Read the model definition and answer for the solid it produces. Units are mm, in the model's axes. A direction names the side the tool comes from. Give positions to 0.01 mm unless a question says otherwise; leave off trailing zeros. Order: outer loops, then holes, each group sorted by start corner. A loop starts at its lowest first (then second) coordinate and runs counter-clockwise, first axis right, second up. Notation, with made-up numbers: (78, -19.75) - (89, -19.75) arc R22 ccw to (89, 8.25) - close; hole circle Ø10 at (37.5, -33). An arc over 180 degrees is marked (long way). Write item = value, one per line.
```python
from build123d import *

# Parameters (mm, degrees)
SKETCH1_R           = 1.5
BOSS_EXTRUDE1_DEPTH = 3
SKETCH2_W           = 26.5
SKETCH2_H           = 13.12704922
BOSS_EXTRUDE2_DEPTH = 3
SKETCH3_R           = 1.5
CUT_EXTRUDE1_DEPTH  = 10
SKETCH4_R           = 1.5
CUT_EXTRUDE2_DEPTH  = 10
BOSS_EXTRUDE4_START = -4
SKETCH6_R           = 1.5
SKETCH6_W           = 26.5
SKETCH6_H           = 25.74798773
BOSS_EXTRUDE4_DEPTH = 4
SKETCH9_R           = 1.5
CUT_EXTRUDE3_DEPTH  = 6
CUT_EXTRUDE4_DEPTH  = 14
SKETCH11_R          = 1.5
CUT_EXTRUDE5_DEPTH  = 14
SKETCH12_W          = 9.439157555
SKETCH12_H          = 13.291874924
CUT_EXTRUDE6_DEPTH  = 10
BOSS_EXTRUDE5_START = -6
SKETCH14_R          = 1.5
SKETCH14_R_2        = 1.624180029
SKETCH14_W          = 10
SKETCH14_H          = 12.873993865
SKETCH14_R_3        = 1.585240738
BOSS_EXTRUDE5_DEPTH = 6
SKETCH15_W          = 23.25
SKETCH15_H          = 10.234024539
CUT_EXTRUDE7_DEPTH  = 3
FILLET2_R           = 10
FILLET4_R           = 10
SKETCH16_W          = 26.5
SKETCH16_H          = 25.74798773
SKETCH16_H_2        = 10.370938511
SKETCH16_W_2        = 9.439157555
SKETCH16_H_3        = 13.291874924
BOSS_EXTRUDE6_DEPTH = 4
FILLET5_R           = 10


with BuildPart() as part:
    # Sketch1 → Boss-Extrude1 (new body)
    with BuildSketch(Plane(origin=(0, 0, 0), x_dir=(1, 0, 0), z_dir=(0, 1, 0))):
        Polygon((-5, -5), (41.5, -5), (41.5, 64.6), (31.5, 64.6), (-5, 56.73), align=None)
        Polygon((31.5, 54.48), (31.5, 5.234024539), (5, 5.234024539), (5, 56.73), align=None, mode=Mode.SUBTRACT)
        with Locations(Location((0, 0, 0), (0, 0, 270))):
            Circle(SKETCH1_R, mode=Mode.SUBTRACT)
        with Locations(Location((0, 51.73, 0), (0, 0, 270))):
            Circle(SKETCH1_R, mode=Mode.SUBTRACT)
        with Locations(Location((36.5, 59.6, 0), (0, 0, 270))):
            Circle(SKETCH1_R, mode=Mode.SUBTRACT)
        with Locations(Location((36.5, 11.18, 0), (0, 0, 270))):
            Circle(SKETCH1_R, mode=Mode.SUBTRACT)
        with Locations(Location((36.5, 49.6, 0), (0, 0, 270))):
            Circle(SKETCH1_R, mode=Mode.SUBTRACT)
    extrude(amount=BOSS_EXTRUDE1_DEPTH)

    # Sketch2 → Boss-Extrude2 (add)
    with BuildSketch(Plane(origin=(0, 3, 0), x_dir=(1, 0, 0), z_dir=(0, 1, 0))):
        with Locations((18.25, 37.545536879)):
            Rectangle(SKETCH2_W, SKETCH2_H)
        Polygon((5, 56.73), (5, 49.867078553), (31.5, 54.48), align=None)
    extrude(amount=-BOSS_EXTRUDE2_DEPTH)

    # Sketch3 → Cut-Extrude1 (cut)
    with BuildSketch(Plane(origin=(0, 3, 0), x_dir=(1, 0, 0), z_dir=(0, 1, 0))):
        with Locations(Location((10, 0, 0), (0, 0, 270))):
            Circle(SKETCH3_R)
    extrude(amount=-CUT_EXTRUDE1_DEPTH, mode=Mode.SUBTRACT)

    # Sketch4 → Cut-Extrude2 (cut)
    with BuildSketch(Plane(origin=(0, 3, 0), x_dir=(1, 0, 0), z_dir=(0, 1, 0))):
        with Locations(Location((0, 8, 0), (0, 0, 270))):
            Circle(SKETCH4_R)
    extrude(amount=-CUT_EXTRUDE2_DEPTH, mode=Mode.SUBTRACT)

    # Sketch6 → Boss-Extrude4 (add)
    # profile 1 of 3: a face of its own
    with BuildSketch(Plane(origin=(0, 3, 0), x_dir=(1, 0, 0), z_dir=(0, 1, 0)).offset(BOSS_EXTRUDE4_START)):
        Polygon((238, 64.6), (41.5, 64.6), (41.5, 29.8), (121.5, 49.6), (201.5, 29.8), (201.5, 56.73), align=None)
    # profile 2 of 3: a face of its own
    with BuildSketch(Plane(origin=(0, 3, 0), x_dir=(1, 0, 0), z_dir=(0, 1, 0)).offset(BOSS_EXTRUDE4_START)):
        Polygon((31.5, 64.6), (-5, 56.73), (-5, -5), (41.5, -5), (41.5, 29.8), (41.5, 64.6), align=None)
        with Locations(Location((0, 0, 0), (0, 0, 270))):
            Circle(SKETCH6_R, mode=Mode.SUBTRACT)
        with Locations(Location((10, 0, 0), (0, 0, 270))):
            Circle(SKETCH6_R, mode=Mode.SUBTRACT)
        with Locations(Location((0, 8, 0), (0, 0, 270))):
            Circle(SKETCH6_R, mode=Mode.SUBTRACT)
        with Locations(Location((36.5, 11.18, 0), (0, 0, 270))):
            Circle(SKETCH6_R, mode=Mode.SUBTRACT)
        with Locations((18.25, 18.108018404)):
            Rectangle(SKETCH6_W, SKETCH6_H, mode=Mode.SUBTRACT)
        Polygon((31.5, 44.109061489), (5, 44.109061489), (5, 49.867078553), (31.5, 54.48), align=None, mode=Mode.SUBTRACT)
        with Locations(Location((0, 51.73, 0), (0, 0, 270))):
            Circle(SKETCH6_R, mode=Mode.SUBTRACT)
        with Locations(Location((36.5, 49.6, 0), (0, 0, 270))):
            Circle(SKETCH6_R, mode=Mode.SUBTRACT)
        with Locations(Location((36.5, 59.6, 0), (0, 0, 270))):
            Circle(SKETCH6_R, mode=Mode.SUBTRACT)
    # profile 3 of 3: a face of its own
    with BuildSketch(Plane(origin=(0, 3, 0), x_dir=(1, 0, 0), z_dir=(0, 1, 0)).offset(BOSS_EXTRUDE4_START)):
        Polygon((248, 64.6), (238, 64.6), (201.5, 56.73), (201.5, -5), (248, -5), align=None)
        with Locations(Location((206.5, 8, 0), (0, 0, 270))):
            Circle(SKETCH6_R, mode=Mode.SUBTRACT)
        with Locations(Location((206.5, 0, 0), (0, 0, 270))):
            Circle(SKETCH6_R, mode=Mode.SUBTRACT)
        with Locations(Location((216.5, 0, 0), (0, 0, 270))):
            Circle(SKETCH6_R, mode=Mode.SUBTRACT)
        with Locations(Location((243, 11.18, 0), (0, 0, 270))):
            Circle(SKETCH6_R, mode=Mode.SUBTRACT)
        with Locations(Location((243, 49.6, 0), (0, 0, 270))):
            Circle(SKETCH6_R, mode=Mode.SUBTRACT)
        with Locations(Location((243, 59.6, 0), (0, 0, 270))):
            Circle(SKETCH6_R, mode=Mode.SUBTRACT)
        with Locations(Location((206.5, 51.73, 0), (0, 0, 270))):
            Circle(SKETCH6_R, mode=Mode.SUBTRACT)
        with Locations((224.75, 18.108018404)):
            Rectangle(SKETCH6_W, SKETCH6_H, mode=Mode.SUBTRACT)
        Polygon((238, 54.48), (238, 44.109061489), (211.5, 44.109061489), (211.5, 49.867078553), align=None, mode=Mode.SUBTRACT)
    extrude(amount=BOSS_EXTRUDE4_DEPTH)

    # Sketch9 → Cut-Extrude3 (cut)
    with BuildSketch(Plane(origin=(0, 3, 0), x_dir=(1, 0, 0), z_dir=(0, 1, 0))):
        with Locations(Location((61.5, 49.6, 0), (0, 0, 270))):
            Circle(SKETCH9_R)
        with Locations(Location((181.5, 49.6, 0), (0, 0, 270))):
            Circle(SKETCH9_R)
    extrude(amount=-CUT_EXTRUDE3_DEPTH, mode=Mode.SUBTRACT)

    # Sketch10 → Cut-Extrude4 (cut)
    with BuildSketch(Plane(origin=(0, 3, 0), x_dir=(1, 0, 0), z_dir=(0, 1, 0))):
        Polygon((79.758586054, 59.447076053), (79.758586054, 45.354236602), (102.023308671, 51.934500024), (102.023308671, 55.399132807), align=None)
        Polygon((140.976691329, 51.934500024), (140.976691329, 55.399132807), (163.241413946, 59.447076053), (163.241413946, 45.354236602), align=None)
    extrude(amount=-CUT_EXTRUDE4_DEPTH, mode=Mode.SUBTRACT)

    # Sketch11 → Cut-Extrude5 (cut)
    with BuildSketch(Plane(origin=(0, 3, 0), x_dir=(1, 0, 0), z_dir=(0, 1, 0))):
        with Locations(Location((71.5, 49.6, 0), (0, 0, 270))):
            Circle(SKETCH11_R)
        with Locations(Location((171.5, 49.6, 0), (0, 0, 270))):
            Circle(SKETCH11_R)
    extrude(amount=-CUT_EXTRUDE5_DEPTH, mode=Mode.SUBTRACT)

    # Sketch12 → Cut-Extrude6 (cut)
    with BuildSketch(Plane(origin=(0, 3, 0), x_dir=(1, 0, 0), z_dir=(0, 1, 0))):
        with Locations((193.819806215, 48.516488721)):
            Rectangle(SKETCH12_W, SKETCH12_H)
        with Locations((49.180193786, 48.516488721)):
            Rectangle(SKETCH12_W, SKETCH12_H)
    extrude(amount=-CUT_EXTRUDE6_DEPTH, mode=Mode.SUBTRACT)

    # Sketch14 → Boss-Extrude5 (add)
    # profile 1 of 6: a face of its own
    with BuildSketch(Plane(origin=(0, 3, 0), x_dir=(1, 0, 0), z_dir=(0, 1, 0)).offset(BOSS_EXTRUDE5_START)):
        Polygon((5, 18.108018404), (-5, 18.108018404), (-5, -5), (5, -5), (18.25, -5), (18.25, 5.234024539), (5, 5.234024539), align=None)
        with Locations(Location((0, 0, 0), (0, 0, 270))):
            Circle(SKETCH14_R, mode=Mode.SUBTRACT)
        with Locations(Location((10, 0, 0), (0, 0, 270))):
            Circle(SKETCH14_R, mode=Mode.SUBTRACT)
        with Locations(Location((0, 8, 0), (0, 0, 270))):
            Circle(SKETCH14_R_2, mode=Mode.SUBTRACT)
    # profile 2 of 6: a face of its own
    with BuildSketch(Plane(origin=(0, 3, 0), x_dir=(1, 0, 0), z_dir=(0, 1, 0)).offset(BOSS_EXTRUDE5_START)):
        Polygon((31.5, 5.234024539), (18.25, 5.234024539), (18.25, -5), (31.5, -5), (41.5, -5), (41.5, 5.234024539), align=None)
    # profile 3 of 6: a face of its own
    with BuildSketch(Plane(origin=(0, 3, 0), x_dir=(1, 0, 0), z_dir=(0, 1, 0)).offset(BOSS_EXTRUDE5_START)):
        with Locations((36.5, 11.671021472)):
            Rectangle(SKETCH14_W, SKETCH14_H)
        with Locations(Location((36.5, 11.18, 0), (0, 0, 270))):
            Circle(SKETCH14_R_3, mode=Mode.SUBTRACT)
    # profile 4 of 6: a face of its own
    with BuildSketch(Plane(origin=(0, 3, 0), x_dir=(1, 0, 0), z_dir=(0, 1, 0)).offset(BOSS_EXTRUDE5_START)):
        with Locations((243, 11.671021472)):
            Rectangle(SKETCH14_W, SKETCH14_H)
        with Locations(Location((243, 11.18, 0), (0, 0, 270))):
            Circle(SKETCH14_R, mode=Mode.SUBTRACT)
    # profile 5 of 6: a face of its own
    with BuildSketch(Plane(origin=(0, 3, 0), x_dir=(1, 0, 0), z_dir=(0, 1, 0)).offset(BOSS_EXTRUDE5_START)):
        Polygon((248, -5), (248, 5.234024539), (238, 5.234024539), (224.75, 5.234024539), (224.75, -5), (238, -5), align=None)
    # profile 6 of 6: a face of its own
    with BuildSketch(Plane(origin=(0, 3, 0), x_dir=(1, 0, 0), z_dir=(0, 1, 0)).offset(BOSS_EXTRUDE5_START)):
        Polygon((224.75, -5), (224.75, 5.234024539), (211.5, 5.234024539), (211.5, 18.108018404), (201.5, 18.108018404), (201.5, -5), (211.5, -5), align=None)
        with Locations(Location((206.5, 0, 0), (0, 0, 270))):
            Circle(SKETCH14_R, mode=Mode.SUBTRACT)
        with Locations(Location((216.5, 0, 0), (0, 0, 270))):
            Circle(SKETCH14_R, mode=Mode.SUBTRACT)
        with Locations(Location((206.5, 8, 0), (0, 0, 270))):
            Circle(SKETCH14_R, mode=Mode.SUBTRACT)
    extrude(amount=BOSS_EXTRUDE5_DEPTH)

    # Sketch15 → Cut-Extrude7 (cut)
    with BuildSketch(Plane(origin=(0, -3, 0), x_dir=(-1, 0, 0), z_dir=(0, -1, 0))):
        with Locations((-29.875, 0.117012269)):
            Rectangle(SKETCH15_W, SKETCH15_H)
        with Locations((-236.375, 0.117012269)):
            Rectangle(SKETCH15_W, SKETCH15_H)
    extrude(amount=-CUT_EXTRUDE7_DEPTH, mode=Mode.SUBTRACT)

    # Fillet2
    # the kernel refuses this fillet: 10 mm, written as the material it adds along each edge
    with BuildSketch(Plane(origin=(224.75, 0, 5), x_dir=(1, 0, 0), z_dir=(0, 0, -1)), Plane(origin=(18.25, 0, 5), x_dir=(1, 0, 0), z_dir=(0, 0, -1))) as fillet2_piece_1:
        with BuildLine():
            CenterArc((7.141428429, 10), FILLET2_R, 224.427004001, 45.572995999)
            Line((0, 3), (0, 0))
            Line((0, 0), (7.141428429, 0))
        make_face()
    extrude(amount=10.234024539)
    with BuildSketch(Plane(origin=(238, 0, -5.234024539), x_dir=(0, -1, 0), z_dir=(1, 0, 0)), Plane(origin=(31.5, 0, -5.234024539), x_dir=(0, -1, 0), z_dir=(1, 0, 0))) as fillet2_piece_2:
        with BuildLine():
            CenterArc((10, -7.141428429), FILLET2_R, 134.427004001, 45.572995999)
            Line((0, -7.141428429), (0, 0))
            Line((0, 0), (3, 0))
        make_face()
    extrude(amount=10)

    # Fillet4
    # the kernel refuses this fillet: 10 mm, written as the material it adds along each edge
    with BuildSketch(Plane(origin=(238, -1, -18.108018404), x_dir=(0, -1, 0), z_dir=(1, 0, 0))) as fillet4_piece_1:
        with BuildLine():
            CenterArc((10, 6), FILLET4_R, 180, 36.869897646)
            Line((0, 6), (-0.2, 6))
            Line((-0.2, 6), (-0.2, 0))
            Line((-0.2, 0), (0, -0.2))
            ThreePointArc((0, -0.2), (1, -0.2), (1.84, -0.12))
            Line((1.84, -0.12), (2, 0))
        make_face()
    extrude(amount=10)
    with BuildSketch(Plane(origin=(201.5, -1, -18.108018404), x_dir=(0, 0, -1), z_dir=(1, 0, 0)), Plane(origin=(31.5, -1, -18.108018404), x_dir=(0, 0, -1), z_dir=(1, 0, 0)), Plane(origin=(-5, -1, -18.108018404), x_dir=(0, 0, -1), z_dir=(1, 0, 0))) as fillet4_piece_2:
        with BuildLine():
            CenterArc((6, -10), FILLET4_R, 90, 36.869897646)
            Line((0, -2), (-0.12, -1.84))
            ThreePointArc((-0.12, -1.84), (-0.2, -1), (-0.2, 0))
            Line((-0.2, 0), (0, 0.2))
            Line((0, 0.2), (6, 0.2))
            Line((6, 0.2), (6, 0))
        make_face()
    extrude(amount=10)

    # Sketch16 → Boss-Extrude6 (add)
    with BuildSketch(Plane(origin=(0, 3, 0), x_dir=(1, 0, 0), z_dir=(0, 1, 0))):
        with Locations((18.25, 18.108018404)):
            Rectangle(SKETCH16_W, SKETCH16_H)
        with Locations((224.75, 18.108018404)):
            Rectangle(SKETCH16_W, SKETCH16_H)
        with Locations((18.25, 49.294530745)):
            Rectangle(SKETCH16_W, SKETCH16_H_2)
        with Locations((224.75, 49.294530745)):
            Rectangle(SKETCH16_W, SKETCH16_H_2)
        with Locations((49.180193786, 48.516488721)):
            Rectangle(SKETCH16_W_2, SKETCH16_H_3)
        with Locations((193.819806215, 48.516488721)):
            Rectangle(SKETCH16_W_2, SKETCH16_H_3)
    extrude(amount=-BOSS_EXTRUDE6_DEPTH)

    # Fillet5
    fillet5_edges = [part.edges().sort_by_distance(p)[0] for p in [
        (41.5, 1, -29.8),
        (201.5, 1, -29.8),
    ]]
    fillet(fillet5_edges, radius=FILLET5_R)


solid = part.part
```
1. Determine the mould class of faces 5 (the face through (4, -3, -4)), 6 (the face through (13.51, 0.97, -60.72)), 7 (the face through (199.432, 0.914, -28.063)) for opening direction X: +X half, -X half, draft (parallel to the pull), parting line (faces both ways), or undercut.
Recorded:
face_5 = draft
face_6 = -X half
face_7 = undercut
2. Flat-ended cylindrical pins translate along their axes: pin 1 (1.8 mm diameter, centred on x = 71.5, z = -49.6, fed in from +Y); pin 2 (0.8 mm diameter, centred on x = 234, y = -0.5, fed in from +Z); pin 3 (1 mm diameter, centred on x = 101.5, z = -51.5, fed in from -Y); pin 4 (3 mm diameter, centred on x = 32.5, z = 2, fed in from -Y). Find the tip coordinate at first contact, or state that the pin passes through.
Recorded:
pin_1 = through
pin_2 = -5.23
pin_3 = -1
pin_4 = -0.1
3. For faces 1 (the face through (157.194, 0.972, -40.766)), 2 (the face through (163.241, 1, -52)), 3 (the face through (227.97, -0.8, -0.05)), 4 (the face through (120, -1, -55)), determine the directions among +Z, -Z, +X, -X, +Y, -Y from which every point of the face is accessible in a straight line to the end or side of a thin tool.
Recorded:
face_1 = +Z, +Y, -Y
face_2 = +Y, -Y
face_3 = +Z, -Y
face_4 = -Z, -Y
4. Section A-A (z = -15) is taken. Determine the outline of the cut face in (x, y).
Recorded:
outline = (-5, -3) - (5, -3) - (5, -1) - (31.5, -1) - (31.5, -3) - (41.5, -3) - (41.5, 3) - (-5, 3) - close; (201.5, -3) - (211.5, -3) - (211.5, -1) - (238, -1) - (238, -3) - (248, -3) - (248, 3) - (201.5, 3) - close
5. Straight lines are drawn through the part: L1, parallel to Z at x = 206.5, y = -0.6; L2, parallel to X at y = -2.2, z = -8; L3, parallel to X at y = 0.95, z = -8. For each, find the intervals that lie inside material, in ascending order. Write a range as [from, to].
Recorded:
L1 = [-64.6, -53.23], [-50.23, -9.5], [-6.5, -1.5], [1.5, 5]
L2 = [-5, -1.62], [1.62, 5], [31.5, 41.5], [201.5, 205], [208, 211.5], [238, 248]
L3 = [-5, -1.5], [1.5, 41.5], [201.5, 205], [208, 248]
6. Section B-B (y = 1.5) is taken. Count the separate pieces of the cut face and the enclosed holes in it, and give its area (3 significant figures).
Recorded:
separate_pieces = 1
enclosed_holes = 20
area = 9,820 mm^2
7. Section C-C (z = -41) is taken. Determine the outline of the cut face in (x, y), and give its area (3 significant figures).
Recorded:
outline = (-5, -1) - (86.75, -1) - (86.75, 3) - (-5, 3) - close; (156.25, -1) - (248, -1) - (248, 3) - (156.25, 3) - close
area = 734 mm^2
